CAD build for the part. Positions are in the model's coordinates, mm. A direction names the side the tool comes from. Coordinates: 2 decimals unless noted, no trailing zeros. Use one line per item in the form item = value. Start each with the question number.
from build123d import *

# Parameters (mm, degrees)
BOSS_EXTRUDE1_DEPTH = 1.5
CIRPATTERN1_COUNT   = 8
SKETCH4_W           = 2.7
SKETCH4_H           = 2.7
CUT_EXTRUDE1_DEPTH  = 11.547606867


with BuildPart() as part:
    # Sketch5 → Boss-Extrude1 (new, symmetric)
    with BuildSketch(Plane(origin=(0, 0, 0), x_dir=(1, 0, 0), z_dir=(0, 1, 0))):
        with BuildLine():
            Line((0, 0), (3.342855658, 2.370565581))
            Line((3.342855658, 2.370565581), (3.746267067, 1.80169155))
            Line((3.746267067, 1.80169155), (4.726512919, 2.273109454))
            add(Edge.make_bspline(
                [(4.726512919, 2.273109454), (5.083840243, 2.444954607), (6.11501814, 2.361263688), (7.066052624, 1.805087159)],
                knots=[0, 0, 0, 0, 1, 1, 1, 1], degree=3))
            Line((7.066052624, 1.805087159), (7.108150593, 1.620429032))
            Line((7.108150593, 1.620429032), (7.150245001, 1.435770094))
            add(Edge.make_bspline(
                [(5.244706948, 7.012e-06), (5.641208616, 1.0552e-05), (6.534229602, 0.522356744), (7.150245001, 1.435770094)],
                knots=[0, 0, 0, 0, 1, 1, 1, 1], degree=3))
            Line((5.244706948, 7.012e-06), (4.156995234, -2.698e-06))
            Line((4.156995234, -2.698e-06), (4.039998902, -0.687512906))
            Line((4.039998902, -0.687512906), (0, 0))
        make_face()
    boss_extrude1 = extrude(amount=BOSS_EXTRUDE1_DEPTH, both=True)

    # CirPattern1: Boss-Extrude1 ×8 about axis
    cirpattern1_axis = Axis((0, -1.5, 0), (0, 1, 0))
    for i in range(1, CIRPATTERN1_COUNT):
        add(boss_extrude1.rotate(cirpattern1_axis, i * 360 / CIRPATTERN1_COUNT))

    # Sketch4 → Cut-Extrude1 (cut, through all)
    with BuildSketch(Plane(origin=(0, 1.5, 0), x_dir=(1, 0, 0), z_dir=(0, 1, 0))):
        Rectangle(SKETCH4_W, SKETCH4_H)
    extrude(amount=-CUT_EXTRUDE1_DEPTH, mode=Mode.SUBTRACT)


solid = part.part
1) Probe L1, parallel to Z at x = -3.5, y = 0.55; L2, parallel to X at y = 0.9, z = 4.25; L3, parallel to X at y = -1.3, z = 6. List the from-to ranges inside material, lowest first.
2) 3-axis set-ups, long thin cutter, end or side, ignore diameter. For faces 1 (the face through (4.429, 0.021, 1.552)), 2 (the face through (2.034, 0.021, 4.23)), 3 (the face through (1.552, 0.021, -4.429)): which of +Z, -Z, +X, -X, +Y, -Y reach the whole face in a straight line?
3) Drop flat-ended pins along their axis: P1, Ø0.8, axis at x = 0.5, y = 0.5, coming from the +Z side; P2, Ø1, axis at y = 1, z = -5, coming from the -X side; P3, Ø0.9, axis at y = 0.5, z = -4.5, coming from the +X side. Give the stop position or say it passes through.
Values follow:
q1.L1 = -3.5 to 2.15, 3.5 to 6.21
q1.L2 = -3.98 to -1.49, 0 to 2.04
q1.L3 = -4.05 to -2.98, 0.3 to 2.24
q2.face_1 = +X, +Y, -Y
q2.face_2 = +Y, -Y
q2.face_3 = -Z, +Y, -Y
q3.P1 = 6.72
q3.P2 = -2.35
q3.P3 = 4.1
